The listing builds one solid part. Answer for the finished solid, in the listing's coordinates (mm). A direction names the side the tool comes from. Round coordinates to 2 decimals unless told otherwise and drop trailing zeros. Write each loop counter-clockwise with the first axis right and the second up, starting at its lowest first coordinate (ties: lowest second). Pieces come first, ordered by that corner, then holes. Notation, with made-up numbers: (6, 10.25) -> (39, 10.25) arc R28 cw to (39, 37.25) -> close; hole circle Ø8 at (46.25, 30.25). An arc over 180 degrees is marked (long way). Write each question's results on one line, items separated by ' | '. Start each with the question number.
```python
from build123d import *

# Parameters (mm, degrees)
F0_W      = 110
F0_H      = 60
F1_DEPTH  = 8
F3_DEPTH  = 2
F5_DEPTH  = 2
F6_W      = 6
F6_H      = 56
F7_DEPTH  = 42
F8_W      = 13
F8_H      = 8
F9_DEPTH  = 8
F10_R     = 3.99999
F11_R     = 2
F12_R     = 1.725
F13_DEPTH = 6
F12_R_2   = 3.5
F14_DEPTH = 3
F17_R     = 5.5
F18_DEPTH = 8
F19_R     = 1.725
F20_DEPTH = 8
F19_R_2   = 14
F21_DEPTH = 55
F22_R     = 32


# Not quite as in the source:
# - a fillet or chamfer is up to 0.001 mm smaller than in the source, because OpenCascade refuses the exact size


with BuildPart() as f1:
    # F0 (on Top) → F1 (new body)
    with BuildSketch(Plane.XY):
        with Locations((55, 30)):
            Rectangle(F0_W, F0_H)
    extrude(amount=F1_DEPTH)

    # F2 (on face) → F3 (join)
    with BuildSketch(Plane.XZ):
        Polygon((0, 8), (110, 8), (110, 50), (102, 50), (60, 16), (0, 16), align=None)
    extrude(amount=-F3_DEPTH)

    # F4 (on face) → F5 (join)
    with BuildSketch(Plane(origin=(0, 60, 0), x_dir=(-1, 0, 0), z_dir=(0, 1, 0))):
        Polygon((-110, 50), (-110, 8), (0, 8), (0, 16), (-60, 16), (-102, 50), align=None)
    extrude(amount=-F5_DEPTH)

    # F6 (on face) → F7 (join)
    with BuildSketch(Plane.XY.offset(8)):
        with Locations((107, 30)):
            Rectangle(F6_W, F6_H)
    extrude(amount=F7_DEPTH)

    # F8 (on face) → F9 (cut)
    with BuildSketch(Plane.XY.offset(8)):
        with Locations((6.5, 30)):
            Rectangle(F8_W, F8_H)
    extrude(amount=-F9_DEPTH, mode=Mode.SUBTRACT)

    # F10 (radius 4 in the source; OpenCascade refuses exactly that, so slightly less here)
    f10_edges = [f1.edges().sort_by_distance(p)[0] for p in [
        (102, 59, 50),
        (102, 1, 50),
        (0, 60, 8),
        (0, 34, 4),
        (0, 26, 4),
        (13, 26, 4),
        (13, 34, 4),
        (0, 0, 8),
    ]]
    fillet(f10_edges, radius=F10_R)

    # F11
    f11_edges = [f1.edges().sort_by_distance(p)[0] for p in [
        (52.267947, 58, 8),
        (52.267947, 2, 8),
        (110, 0, 25),
        (110, 60, 25),
        (104, 2, 29),
        (104, 58, 29),
        (104, 30, 8),
    ]]
    fillet(f11_edges, radius=F11_R)

    # F12 (on face) → F13 (cut)
    with BuildSketch(Plane.YZ.offset(110)):
        with Locations((20, 37.5)):
            Circle(F12_R)
        with Locations((40, 22.5)):
            Circle(F12_R)
        with Locations((20, 22.5)):
            Circle(F12_R)
        with Locations((40, 37.5)):
            Circle(F12_R)
    extrude(amount=-F13_DEPTH, mode=Mode.SUBTRACT)


with BuildPart() as f14:
    # F12 (on face) → F14 (new body)
    with BuildSketch(Plane.YZ.offset(110)):
        with Locations((20, 22.5)):
            Circle(F12_R_2)
        with Locations((20, 22.5)):
            Circle(F12_R, mode=Mode.SUBTRACT)
    extrude(amount=-F14_DEPTH)


with BuildPart() as f14b:
    # F12 (on face) → F14, piece 2 (new body)
    with BuildSketch(Plane.YZ.offset(110)):
        with Locations((40, 22.5)):
            Circle(F12_R_2)
        with Locations((40, 22.5)):
            Circle(F12_R, mode=Mode.SUBTRACT)
    extrude(amount=-F14_DEPTH)


with BuildPart() as f14c:
    # F12 (on face) → F14, piece 3 (new body)
    with BuildSketch(Plane.YZ.offset(110)):
        with Locations((40, 37.5)):
            Circle(F12_R_2)
        with Locations((40, 37.5)):
            Circle(F12_R, mode=Mode.SUBTRACT)
    extrude(amount=-F14_DEPTH)


with BuildPart() as f14d:
    # F12 (on face) → F14, piece 4 (new body)
    with BuildSketch(Plane.YZ.offset(110)):
        with Locations((20, 37.5)):
            Circle(F12_R_2)
        with Locations((20, 37.5)):
            Circle(F12_R, mode=Mode.SUBTRACT)
    extrude(amount=-F14_DEPTH)


with BuildPart() as f14d_1:
    # F15: moved
    add(f14d.part.moved(Location((-4, 0, 0))))


with BuildPart() as f14c_1:
    # F15: moved
    add(f14c.part.moved(Location((-4, 0, 0))))


with BuildPart() as f14b_1:
    # F15: moved
    add(f14b.part.moved(Location((-4, 0, 0))))


with BuildPart() as f14_1:
    # F15: moved
    add(f14.part.moved(Location((-4, 0, 0))))


with BuildPart() as f1_1:
    add(f1.part)

    # F16: cut F14d, F14c, F14b, F14
    add(f14d_1.part, mode=Mode.SUBTRACT)
    add(f14c_1.part, mode=Mode.SUBTRACT)
    add(f14b_1.part, mode=Mode.SUBTRACT)
    add(f14_1.part, mode=Mode.SUBTRACT)

    # F17 (on face) → F18 (cut)
    with BuildSketch(Plane(origin=(0, 0, 0), x_dir=(1, 0, 0), z_dir=(0, 0, -1))):
        with Locations((91, -30)):
            Circle(F17_R)
    extrude(amount=-F18_DEPTH, mode=Mode.SUBTRACT)

    # F19 (on face) → F20 (cut)
    with BuildSketch(Plane.XY.offset(8)):
        with Locations((91, 37.6)):
            Circle(F19_R)
        with Locations((91, 22.4)):
            Circle(F19_R)
    extrude(amount=-F20_DEPTH, mode=Mode.SUBTRACT)

    # F19 (on face) → F21 (cut)
    with BuildSketch(Plane.XY.offset(8)):
        with Locations((91, 30)):
            Circle(F19_R_2)
        with Locations((91, 22.4)):
            Circle(F19_R, mode=Mode.SUBTRACT)
        with Locations((83.4, 30)):
            Circle(F19_R, mode=Mode.SUBTRACT)
        with Locations((91, 37.6)):
            Circle(F19_R, mode=Mode.SUBTRACT)
        with Locations((98.6, 30)):
            Circle(F19_R, mode=Mode.SUBTRACT)
        with Locations((-18, 77.4)):
            Circle(F19_R)
        with Locations((-77.4, -18)):
            Circle(F19_R)
        with Locations((18, -77.4)):
            Circle(F19_R)
        with Locations((98.6, 30)):
            Circle(F19_R)
    extrude(amount=F21_DEPTH, mode=Mode.SUBTRACT)

    # F22
    f22_edges = [f1_1.edges().sort_by_distance(p)[0] for p in [
        (60, 59, 16),
        (60, 1, 16),
    ]]
    fillet(f22_edges, radius=F22_R)


solid = f1_1.part
```
Q1. Determine the mould class of faces 1 (the flat face through (68, 60, 14)), 2 (the flat face through (107, 30, 50)), 3 (the flat face through (104, 14, 30)) for opening direction Y: pulls with the +Y half, pulls with the -Y half, needs draft (parallel to the pull), parting line crosses it, or undercut.
Q2. For faces 4 (the cylindrical face through (85.505, 29.758, 3.944)), 5 (the flat face through (70, 58, 21)), 6 (the cylindrical face through (105, 20, 41)), 7 (the flat face through (0, 13, 4)), 8 (the flat face through (6, 34, 4)), determine the directions among +Z, -Z, +X, -X, +Y, -Y from which every point of the face is accessible in a straight line to the end or side of a thin tool.
Q3. The part is cut by section B-B, the plane y = 32.5. Write down the section's boundary in (x, z), then the cut area to 3 significant figures.
Q4. The part is cut by section A-A, the plane z = 4. State how many separate pieces and enclosed holes the cut face has, then the cut area to 3 significant figures.
Q5. Each of these flat-tipped pins is pushed along its axis until it touches: pin 1 (12 mm diameter, centred on x = 87.5, y = 35, fed in from +Z); pin 2 (1.6 mm diameter, centred on x = 29.5, y = 59.5, fed in from +Z); pin 3 (4 mm diameter, centred on y = 40, z = 22.5, fed in from -X). Where does it stop, or does it pass through?
Q6. Find the intervals of material crossed by line 1 (Z direction, x = 105.5, y = 40); line 2 (Y direction, x = 91, z = 4.75) (3 decimals); line 3 (Z direction, x = 108, y = 20) (3 decimals), in increasing order.
Q7. The part is cut by section C-C, the plane x = 91. Write down the section's boundary in (y, z) (3 decimals).
Answers follow:
1) face 1: pulls with the +Y half | face 2: needs draft | face 3: undercut
2) face 4: +Z, -Z | face 5: +Z, -X | face 6: -X | face 7: +Z, -Z, -X, +Y, -Y | face 8: +Z, -Z, -X
3) outline: (12.12, 0) -> (86.1, 0) -> (86.1, 8) -> (12.12, 8) -> close; (95.9, 0) -> (110, 0) -> (110, 50) -> (104.77, 50) -> (104.77, 8) -> (95.9, 8) -> close | area: 924 mm^2
4) separate pieces: 1 | enclosed holes: 3 | area: 6,370 mm^2
5) pin 1: z = 8 | pin 2: z = 16 | pin 3: x = 106
6) line 1: 0 to 19, 26 to 34, 41 to 50 | line 2: 0 to 20.675, 24.125 to 24.5, 35.5 to 35.875, 39.325 to 60 | line 3: 0 to 20.775, 24.225 to 35.775, 39.225 to 50
7) outline: (0, 0) -> (20.675, 0) -> (20.675, 8) -> (4, 8) arc R2 cw to (2, 10) -> (2, 41.095) -> (0, 41.095) -> close; (24.125, 0) -> (24.5, 0) -> (24.5, 8) -> (24.125, 8) -> close; (35.5, 0) -> (35.875, 0) -> (35.875, 8) -> (35.5, 8) -> close; (39.325, 0) -> (60, 0) -> (60, 41.095) -> (58, 41.095) -> (58, 10) arc R2 cw to (56, 8) -> (39.325, 8) -> close
